The listing builds one solid part. Answer for the finished solid, in the listing's coordinates (mm). A direction names the side the tool comes from. Round coordinates to 2 decimals unless told otherwise and drop trailing zeros. Order: outer loops, then holes, each group sorted by start corner. A loop starts at its lowest first (then second) coordinate and runs counter-clockwise, first axis right, second up. Notation, with made-up numbers: (21.25, 27.5) - (35.25, 27.5) arc R24 cw to (35.25, 60.5) - close; hole circle Ø4 at (-10, -25.5). An arc over 180 degrees is marked (long way). Use CSV: the item, a comma, the result in double quotes. Start each with the question number.
Item 1: Determine the mould class of faces 1 (the flat face through (34, 2, 32.21)), 2 (the flat face through (0, 2, 41)), 3 (the flat face through (42, 2, 0)), 4 (the cylindrical face through (76.05, 1.57, 4.75)) for opening direction Z: +Z half, -Z half, draft (parallel to the pull), parting line (faces both ways), or undercut.
Item 2: Find section C-C, the plane y = 1.6. Give the vertices of the cut face in (x, z).
Item 3: Find section A-A, the plane z = 57. Give the vertices of the cut face in (x, y) (3 decimals).
Item 4: Straight lines are drawn through the part: line 1 along Z through (x, y) = (39, 2.65); line 2 along X through (y, z) = (1.25, 4); line 3 along X through (y, z) = (1.3, 39). For each, find the intervals that lie inside material, in ascending order. Write a range as [from, to].
Item 5: For faces 5 (the flat face through (42, 2, 80)), 6 (the flat face through (34, 2, 10.21)), determine the directions among +Z, -Z, +X, -X, +Y, -Y from which every point of the face is accessible in a straight line to the end or side of a thin tool.
Item 6: Find section D-D, the plane z = 69. Give the vertices of the cut face in (x, y) (3 decimals).
Item 7: Flat-ended cylindrical pins translate along their axes: P1, Ø1.6, axis at y = 2, z = 53.5, coming from the -X side; P2, Ø2.5, axis at x = 7.5, z = 4, coming from the -Y side. Find the tip coordinate at first contact, or state that the pin passes through.
Item 8: Find section B-B, the plane x = 59. Give the vertices of the cut face in (y, z) (3 decimals), plus the area to 3 significant figures.
```python
from build123d import *

# Parameters (mm, degrees)
SKETCH1_W           = 85
SKETCH1_H           = 80
SKETCH1_R           = 1.63195
SKETCH1_R_2         = 6.5
SKETCH1_W_2         = 52
SKETCH1_H_2         = 22
BOSS_EXTRUDE1_DEPTH = 3.175


with BuildPart() as part:
    # Sketch1 → Boss-Extrude1 (new body)
    with BuildSketch(Plane(origin=(0, 0, 0), x_dir=(1, 0, 0), z_dir=(0, 1, 0))):
        with Locations((42.5, -40)):
            Rectangle(SKETCH1_W, SKETCH1_H)
        with Locations(Location((7.5, -4, 0), (0, 0, 270))):
            Circle(SKETCH1_R, mode=Mode.SUBTRACT)
        with Locations(Location((7.5, -69, 0), (0, 0, 270))):
            Circle(SKETCH1_R, mode=Mode.SUBTRACT)
        with Locations(Location((77.5, -69, 0), (0, 0, 270))):
            Circle(SKETCH1_R, mode=Mode.SUBTRACT)
        with Locations(Location((77.5, -4, 0), (0, 0, 270))):
            Circle(SKETCH1_R, mode=Mode.SUBTRACT)
        with Locations(Location((76, -39, 0), (0, 0, 270))):
            Circle(SKETCH1_R_2, mode=Mode.SUBTRACT)
        with Locations((34, -49.95)):
            Rectangle(SKETCH1_W_2, SKETCH1_H_2, mode=Mode.SUBTRACT)
        with Locations((34, -21.21)):
            Rectangle(SKETCH1_W_2, SKETCH1_H_2, mode=Mode.SUBTRACT)
    extrude(amount=BOSS_EXTRUDE1_DEPTH)


solid = part.part
```
Worked out:
1,face 1,"undercut"
1,face 2,"draft"
1,face 3,"-Z half"
1,face 4,"undercut"
2,outline,"(0, 0) - (85, 0) - (85, 80) - (0, 80) - close; hole circle Ø3.26 at (7.5, 4); hole circle Ø3.26 at (7.5, 69); hole (8, 10.21) - (60, 10.21) - (60, 32.21) - (8, 32.21) - close; hole (8, 38.95) - (60, 38.95) - (60, 60.95) - (8, 60.95) - close; hole circle Ø13 at (76, 39); hole circle Ø3.26 at (77.5, 4); hole circle Ø3.26 at (77.5, 69)"
3,outline,"(0, 0) - (8, 0) - (8, 3.175) - (0, 3.175) - close; (60, 0) - (85, 0) - (85, 3.175) - (60, 3.175) - close"
4,line 1,"z = [0, 10.21], [32.21, 38.95], [60.95, 80]"
4,line 2,"x = [0, 5.87], [9.13, 75.87], [79.13, 85]"
4,line 3,"x = [0, 8], [60, 69.5], [82.5, 85]"
5,face 5,"+Z, +X, -X, +Y, -Y"
5,face 6,"+Y, -Y"
6,outline,"(0, 0) - (5.868, 0) - (5.868, 3.175) - (0, 3.175) - close; (9.132, 0) - (75.868, 0) - (75.868, 3.175) - (9.132, 3.175) - close; (79.132, 0) - (85, 0) - (85, 3.175) - (79.132, 3.175) - close"
7,P1,"stops at x = 0"
7,P2,"passes through"
8,outline,"(0, 0) - (3.175, 0) - (3.175, 10.21) - (0, 10.21) - close; (0, 32.21) - (3.175, 32.21) - (3.175, 38.95) - (0, 38.95) - close; (0, 60.95) - (3.175, 60.95) - (3.175, 80) - (0, 80) - close"
8,area,"114 mm²"
